For this review, take the finished solid that the model builds, in its own axes (mm). Coordinates: 2 decimals unless noted, no trailing zeros. Loops run counter-clockwise (first coordinate to the right, second up) from the corner with the lowest first, then second, coordinate; pieces in that order, holes last. Notation, with made-up numbers: (16, 49.5) - (50, 49.5) arc R33 cw to (50, 82.5) - close; hole circle Ø2 at (64, 33.5). An arc over 180 degrees is marked (long way). Answer as a JSON object with one key per item and string values. Group by question number.
Item 1: We need section A-A (x = -1.8). Give the boundary of the cut face in (y, z), then the cut area to 3 significant figures.
Item 2: We need section C-C (z = -11). Give the boundary of the cut face in (x, y), then the cut area to 3 significant figures.
Item 3: To check wall thickness, follow line 1 (Y direction, x = -0.5, z = -11.5); line 2 (Y direction, x = -2.7, z = 10); line 3 (Z direction, x = -0.35, y = 14.5). State the ranges of each line that lie inside material, in increasing order.
Item 4: We need section D-D (z = 1). Give the boundary of the cut face in (x, y), then the cut area to 3 significant figures.
Item 5: Mouldability with a two-part tool opening along Y and no side actions: class faces 1 (the flat face through (-3, -5, 0)), 2 (the flat face through (-1.48, -5.91, -13.33)) as released by +Y, released by -Y, zero draft, split by the parting line, or undercut.
Item 6: We need section B-B (y = -9). Give the boundary of the cut face in (x, z), then the cut area to 3 significant figures.
Item 7: Clearance check with flat-ended pins moving along their axes: pin 1 (1.5 mm diameter, centred on x = -2, y = 16, fed in from -Z); pin 2 (1.5 mm diameter, centred on x = -2, z = 0.5, fed in from -Y); pin 3 (1 mm diameter, centred on x = -1.5, z = -8.5, fed in from -Y). State where each tip first meets the part, or that it passes through.
from build123d import *

# Parameters (mm, degrees)
SKETCH_5_R      = 24
EXTRUDE_1_DEPTH = 3


with BuildPart() as part:
    # Эскиз5 → Бобышка-Вытянуть1 (new body)
    with BuildSketch(Plane.ZY):
        Circle(SKETCH_5_R)
        with BuildLine():
            Line((5.5, 18.708286934), (0, 6.121683557))
            Line((0, 6.121683557), (-5.5, 18.708286934))
            ThreePointArc((-5.5, 18.708286934), (0, 19.5), (5.5, 18.708286934))
        make_face(mode=Mode.SUBTRACT)
        with BuildLine():
            Line((10.076621897, 16.694660558), (3, 0.5))
            Line((3, 0.5), (-3, 0.5))
            Line((-3, 0.5), (-10.076621897, 16.694660558))
            ThreePointArc((-10.076621897, 16.694660558), (-13.01736824, 14.518888529), (-15.5, 11.832159566))
            Line((-15.5, 11.832159566), (-7, -8.016467208))
            Line((-7, -8.016467208), (-3, -0.5))
            Line((-3, -0.5), (3, -0.5))
            Line((3, -0.5), (7, -8.016467208))
            Line((7, -8.016467208), (15.5, 11.832159566))
            ThreePointArc((15.5, 11.832159566), (13.01736824, 14.518888529), (10.076621897, 16.694660558))
        make_face(mode=Mode.SUBTRACT)
        with BuildLine():
            Line((0, -6.5), (5.5, -18.708286934))
            ThreePointArc((5.5, -18.708286934), (0, -19.5), (-5.5, -18.708286934))
            Line((-5.5, -18.708286934), (0, -6.5))
        make_face(mode=Mode.SUBTRACT)
        with BuildLine():
            Line((8.30458122, -17.64324037), (18.5, 6.164414003))
            ThreePointArc((18.5, 6.164414003), (17.925470573, -7.676425257), (8.30458122, -17.64324037))
        make_face(mode=Mode.SUBTRACT)
        with BuildLine():
            Line((-8.30458122, -17.64324037), (-18.5, 6.164414003))
            ThreePointArc((-18.5, 6.164414003), (-17.925470573, -7.676425257), (-8.30458122, -17.64324037))
        make_face(mode=Mode.SUBTRACT)
    extrude(amount=EXTRUDE_1_DEPTH)


solid = part.part
Check sheet entries:
{
 "1": {"outline": "circle Ø48 at (0, 0); hole (-18.71, -5.5) - (-6.5, 0) - (-18.71, 5.5) arc R19.5 ccw to start; hole (-17.64, -8.3) arc R19.5 ccw to (6.16, -18.5) - close; hole (-17.64, 8.3) - (6.16, 18.5) arc R19.5 ccw to start; hole (-8.02, -7) - (11.83, -15.5) arc R19.5 ccw to (16.69, -10.08) - (0.5, -3) - (0.5, 3) - (16.69, 10.08) arc R19.5 ccw to (11.83, 15.5) - (-8.02, 7) - (-0.5, 3) - (-0.5, -3) - close; hole (6.12, 0) - (18.71, -5.5) arc R19.5 ccw to (18.71, 5.5) - close", "area": "1,200 mm2"},
 "2": {"outline": "(-3, -21.33) - (0, -21.33) - (0, -16.1) - (-3, -16.1) - close; (-3, -11.35) - (0, -11.35) - (0, 1.32) - (-3, 1.32) - close; (-3, 16.1) - (0, 16.1) - (0, 21.33) - (-3, 21.33) - close", "area": "69.4 mm2"},
 "3": {"line 1": "y = -21.07 to -15.75, -10.18 to 2.49, 15.75 to 21.07", "line 2": "y = -21.82 to -16.74, -13.68 to -1.01, 16.52 to 21.82", "line 3": "z = -19.12 to -13.04, -9.12 to -3.66, 3.66 to 9.12, 13.04 to 19.12"},
 "4": {"outline": "(-3, -23.98) - (0, -23.98) - (0, -19.47) - (-3, -19.47) - close; (-3, -8.72) - (0, -8.72) - (0, -0.5) - (-3, -0.5) - close; (-3, 0.5) - (0, 0.5) - (0, 8.41) - (-3, 8.41) - close; (-3, 19.47) - (0, 19.47) - (0, 23.98) - (-3, 23.98) - close", "area": "75.4 mm2"},
 "5": {"face 1": "zero draft", "face 2": "undercut"},
 "6": {"outline": "(-3, -22.25) - (0, -22.25) - (0, -17.3) - (-3, -17.3) - close; (-3, -12.01) - (0, -12.01) - (0, -1.13) - (-3, -1.13) - close; (-3, 1.13) - (0, 1.13) - (0, 12.01) - (-3, 12.01) - close; (-3, 17.3) - (0, 17.3) - (0, 22.25) - (-3, 22.25) - close", "area": "95.0 mm2"},
 "7": {"pin 1": "stops at z = -18.53", "pin 2": "stops at y = -24", "pin 3": "stops at y = -22.63"}
}
